Verification items for the finished model (mm, model axes). Face numbers are marked on the shaded views. A direction names the side the tool comes from. Give positions to 0.01 mm unless a question says otherwise; leave off trailing zeros. Order: outer loops, then holes, each group sorted by start corner. A loop starts at its lowest first (then second) coordinate and runs counter-clockwise, first axis right, second up. Notation, with made-up numbers: M 80,-29.5 L 119,-29.5 A24 cw 119,-8.5 Z; hole C 68,72.25 d8. An arc over 180 degrees is marked long. Answer as a JSON object with one key per item and string values.
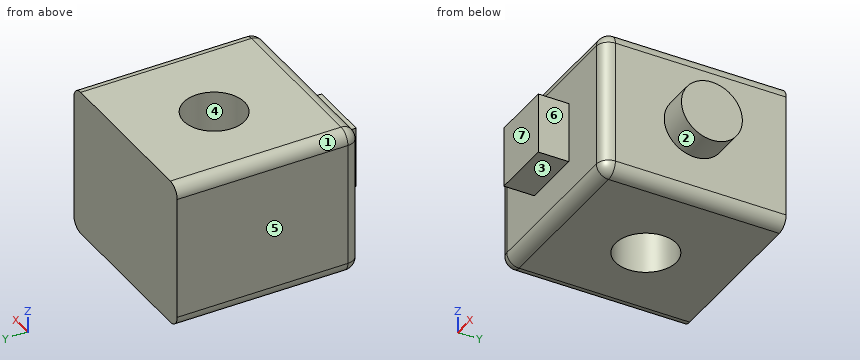
```python
from build123d import *

# Parameters (mm, degrees)
F0_W     = 76.2
F0_H     = 61.731871
F1_DEPTH = 76.2
F4_R     = 12.695575
F5_DEPTH = 12.7
F7_W     = 25.4
F7_H     = 25.4
F8_DEPTH = 12.7
F10_D    = 25.4
F11_R    = 5.08
F12_R    = 5.08
F13_R    = 5.08
F14_R    = 5.08


with BuildPart() as f1:
    # F0 (on Front) → F1 (new body)
    with BuildSketch(Plane.XZ):
        with Locations((38.1, 30.865935)):
            Rectangle(F0_W, F0_H)
    extrude(amount=F1_DEPTH)

    # F4 (on face) → F5 (join)
    with BuildSketch(Plane.YZ.offset(76.2)):
        with Locations((-38.1, 30.42659)):
            Circle(F4_R)
    extrude(amount=F5_DEPTH)

    # F7 (on face) → F8 (join)
    with BuildSketch(Plane.XZ.offset(76.2)):
        with Locations((38.1, 30.749847)):
            Rectangle(F7_W, F7_H)
    extrude(amount=F8_DEPTH)

    # F10 (through all)
    with Locations(Plane.XY.offset(61.731871)):
        with Locations((36.42799, -35.96206)):
            Hole(F10_D / 2)

    # F11
    f11_edges = [f1.edges().sort_by_distance(p)[0] for p in [
        (38.1, -76.2, 61.731871),
    ]]
    fillet(f11_edges, radius=F11_R)

    # F12
    f12_edges = [f1.edges().sort_by_distance(p)[0] for p in [
        (76.2, -35.56, 61.731871),
    ]]
    fillet(f12_edges, radius=F12_R)

    # F13
    f13_edges = [f1.edges().sort_by_distance(p)[0] for p in [
        (0, -35.56, 61.731871),
    ]]
    fillet(f13_edges, radius=F13_R)

    # F14
    f14_edges = [f1.edges().sort_by_distance(p)[0] for p in [
        (38.1, -76.2, 0),
    ]]
    fillet(f14_edges, radius=F14_R)


solid = f1.part
```
Q1. Tool access check on the marked faces 1, 2 and 3. Record the directions out of +Z, -Z, +X, -X, +Y, -Y that give a thin tool (end or side, any length) a straight path to the whole face; none if there is none.
Resolved:
{"face 1": "+Z, -X, +Y, -Y", "face 2": "+X", "face 3": "-Z, +X, -X, -Y"}
Q2. Material ranges on L1, parallel to X at y = -66, z = 11; L2, parallel to X at y = -80, z = 28.5; L3, parallel to Y at x = 68, z = 12, recorded low to high.
Resolved:
{"L1": "x = 0 to 76.2", "L2": "x = 25.4 to 50.8", "L3": "y = -76.2 to 0"}
Q3. Section check D-D on z = 24. Record the cut outline in (x, y).
Resolved:
{"outline": "M 0,-71.12 A5.08 ccw 5.08,-76.2 L 25.4,-76.2 L 25.4,-88.9 L 50.8,-88.9 L 50.8,-76.2 L 71.12,-76.2 A5.08 ccw 76.2,-71.12 L 76.2,-49.05 L 88.9,-49.05 L 88.9,-27.15 L 76.2,-27.15 L 76.2,0 L 0,0 Z; hole C 36.43,-35.96 d25.4"}
Q4. Release check for a two-part mould opening along X. For the marked faces 4, 5, 6 and 7 record: +X half, -X half, draft (parallel to the pull), parting line (faces both ways), or undercut.
Resolved:
{"face 4": "undercut", "face 5": "-X half", "face 6": "+X half", "face 7": "draft"}
Q5. Gauge pin test, flat ends, axial feed: pin 1 Ø10 at (x, y) = (30.5, -76.5) entering from +Z; pin 2 Ø6.5 at (y, z) = (-80, 32.5) entering from -X; pin 3 Ø14 at (x, y) = (38.5, -85) entering from -Z; pin 4 Ø23 at (x, y) = (36.43, -35.96) entering from -Z. Record the tip position at first contact, or that the pin passes through.
Resolved:
{"pin 1": "stops at z = 61.72", "pin 2": "stops at x = 25.4", "pin 3": "stops at z = 18.05", "pin 4": "passes through"}
Q6. Section check C-C on x = 11. Record the cut outline in (y, z), then the cut area to 3 significant figures.
Resolved:
{"outline": "M -76.2,5.08 A5.08 ccw -71.12,0 L 0,0 L 0,61.73 L -71.12,61.73 A5.08 ccw -76.2,56.65 Z", "area": "4,690 mm²"}
Q7. Section check A-A on x = 47. Record the cut outline in (y, z), then the cut area to 3 significant figures.
Resolved:
{"outline": "M -88.9,18.05 L -76.2,18.05 L -76.2,5.08 A5.08 ccw -71.12,0 L -43,0 L -43,61.73 L -71.12,61.73 A5.08 ccw -76.2,56.65 L -76.2,43.45 L -88.9,43.45 Z; M -28.92,0 L 0,0 L 0,61.73 L -28.92,61.73 Z", "area": "4,150 mm²"}
Q8. Section check B-B on y = -42.5. Record the cut outline in (x, z), then the cut area to 3 significant figures.
Resolved:
{"outline": "M 0,5.08 A5.08 ccw 5.08,0 L 25.54,0 L 25.54,61.73 L 5.08,61.73 A5.08 ccw 0,56.65 Z; M 47.32,0 L 71.12,0 A5.08 ccw 76.2,5.08 L 76.2,18.52 L 88.9,18.52 L 88.9,42.34 L 76.2,42.34 L 76.2,56.65 A5.08 ccw 71.12,61.73 L 47.32,61.73 Z", "area": "3,640 mm²"}
